Design review of the part built by this model. Coordinates are the model's own, in mm. A direction names the side the tool comes from. Give positions to 0.01 mm unless a question says otherwise; leave off trailing zeros. Loops run counter-clockwise (first coordinate to the right, second up) from the corner with the lowest first, then second, coordinate; pieces in that order, holes last.
from build123d import *

# Parameters (mm, degrees)
ESQUISSE1_R             = 2.05
ESQUISSE1_R_2           = 1.55
ESQUISSE1_R_3           = 3
BOSS_EXTRU_1_DEPTH      = 9
CONG_2_R                = 5
ESQUISSE2_R             = 1.5
ENL_V_MAT_EXTRU_1_DEPTH = 10


with BuildPart() as part:
    # Esquisse1 → Boss.-Extru.1 (new body)
    with BuildSketch(Plane(origin=(0, 0, 0), x_dir=(1, 0, 0), z_dir=(0, 1, 0))):
        Polygon((150, -69), (150, 69), (-149.848840409, 69), (-150, 69), (-150, -69), (-120, -69), (-120, -99), (120, -99), (120, -69), align=None)
        with Locations(Location((-140, 59, 0), (0, 0, 270))):
            Circle(ESQUISSE1_R, mode=Mode.SUBTRACT)
        with Locations(Location((140, 59, 0), (0, 0, 90))):
            Circle(ESQUISSE1_R, mode=Mode.SUBTRACT)
        with Locations(Location((140, -59, 0), (0, 0, 270))):
            Circle(ESQUISSE1_R, mode=Mode.SUBTRACT)
        with Locations(Location((-140, -59, 0), (0, 0, 90))):
            Circle(ESQUISSE1_R, mode=Mode.SUBTRACT)
        with Locations(Location((-48, -83, 0), (0, 0, 270))):
            Circle(ESQUISSE1_R_2, mode=Mode.SUBTRACT)
        with Locations(Location((-104, -83, 0), (0, 0, 270))):
            Circle(ESQUISSE1_R_2, mode=Mode.SUBTRACT)
        with Locations(Location((-48, -64, 0), (0, 0, 270))):
            Circle(ESQUISSE1_R_2, mode=Mode.SUBTRACT)
        with Locations(Location((-104, -64, 0), (0, 0, 270))):
            Circle(ESQUISSE1_R_2, mode=Mode.SUBTRACT)
        with Locations(Location((82.54, -28.63, 0), (0, 0, 270))):
            Circle(ESQUISSE1_R_2, mode=Mode.SUBTRACT)
        with Locations(Location((130.8, -27.36, 0), (0, 0, 270))):
            Circle(ESQUISSE1_R_2, mode=Mode.SUBTRACT)
        with Locations(Location((130.8, 47.57, 0), (0, 0, 270))):
            Circle(ESQUISSE1_R_2, mode=Mode.SUBTRACT)
        with Locations(Location((82.54, 53.92, 0), (0, 0, 270))):
            Circle(ESQUISSE1_R_2, mode=Mode.SUBTRACT)
        with Locations(Location((87.62, 23.44, 0), (0, 0, 270))):
            Circle(ESQUISSE1_R_2, mode=Mode.SUBTRACT)
        with Locations(Location((38, -54, 0), (0, 0, 270))):
            Circle(ESQUISSE1_R_2, mode=Mode.SUBTRACT)
        with Locations(Location((75, -54, 0), (0, 0, 270))):
            Circle(ESQUISSE1_R_2, mode=Mode.SUBTRACT)
        with Locations(Location((75, -91, 0), (0, 0, 270))):
            Circle(ESQUISSE1_R_2, mode=Mode.SUBTRACT)
        with Locations(Location((38, -91, 0), (0, 0, 270))):
            Circle(ESQUISSE1_R_2, mode=Mode.SUBTRACT)
        with Locations(Location((-132.5, 50.5, 0), (0, 0, 270))):
            Circle(ESQUISSE1_R_2, mode=Mode.SUBTRACT)
        with Locations(Location((-132.5, -7.5, 0), (0, 0, 270))):
            Circle(ESQUISSE1_R_2, mode=Mode.SUBTRACT)
        with Locations(Location((-83.5, -7.5, 0), (0, 0, 270))):
            Circle(ESQUISSE1_R_2, mode=Mode.SUBTRACT)
        with Locations(Location((-83.5, 50.5, 0), (0, 0, 270))):
            Circle(ESQUISSE1_R_2, mode=Mode.SUBTRACT)
        with Locations(Location((-55.25, 52, 0), (0, 0, 270))):
            Circle(ESQUISSE1_R_2, mode=Mode.SUBTRACT)
        with Locations(Location((-55.25, -12, 0), (0, 0, 270))):
            Circle(ESQUISSE1_R_2, mode=Mode.SUBTRACT)
        with Locations(Location((55.25, 52, 0), (0, 0, 270))):
            Circle(ESQUISSE1_R_2, mode=Mode.SUBTRACT)
        with Locations(Location((55.25, -12, 0), (0, 0, 270))):
            Circle(ESQUISSE1_R_2, mode=Mode.SUBTRACT)
        with Locations(Location((-24.75, -56.5, 0), (0, 0, 270))):
            Circle(ESQUISSE1_R_2, mode=Mode.SUBTRACT)
        with Locations(Location((24.75, -56.5, 0), (0, 0, 270))):
            Circle(ESQUISSE1_R_2, mode=Mode.SUBTRACT)
        with Locations(Location((27.5, -72.5, 0), (0, 0, 270))):
            Circle(ESQUISSE1_R_3, mode=Mode.SUBTRACT)
        with Locations(Location((85.5, -72.5, 0), (0, 0, 270))):
            Circle(ESQUISSE1_R_3, mode=Mode.SUBTRACT)
        with Locations(Location((-76, -56, 0), (0, 0, 270))):
            Circle(ESQUISSE1_R_3, mode=Mode.SUBTRACT)
        with BuildLine():
            Line((-56, -95.5), (-96, -95.5))
            ThreePointArc((-96, -95.5), (-98.5, -93), (-96, -90.5))
            Line((-96, -90.5), (-56, -90.5))
            ThreePointArc((-56, -90.5), (-53.5, -93), (-56, -95.5))
        make_face(mode=Mode.SUBTRACT)
        with BuildLine():
            Line((-5, 66.5), (5, 66.5))
            ThreePointArc((5, 66.5), (7.5, 64), (5, 61.5))
            Line((5, 61.5), (-5, 61.5))
            ThreePointArc((-5, 61.5), (-7.5, 64), (-5, 66.5))
        make_face(mode=Mode.SUBTRACT)
        with BuildLine():
            Line((-42.5, -35.25), (-42.5, -45.25))
            ThreePointArc((-42.5, -45.25), (-45, -47.75), (-47.5, -45.25))
            Line((-47.5, -45.25), (-47.5, -35.25))
            ThreePointArc((-47.5, -35.25), (-45, -32.75), (-42.5, -35.25))
        make_face(mode=Mode.SUBTRACT)
        with BuildLine():
            Line((42.5, -35.25), (42.5, -45.25))
            ThreePointArc((42.5, -45.25), (45, -47.75), (47.5, -45.25))
            Line((47.5, -45.25), (47.5, -35.25))
            ThreePointArc((47.5, -35.25), (45, -32.75), (42.5, -35.25))
        make_face(mode=Mode.SUBTRACT)
    extrude(amount=BOSS_EXTRU_1_DEPTH)

    # Congé2
    cong_2_edges = [part.edges().sort_by_distance(p)[0] for p in [
        (150, 4.5, -69),
        (150, 4.5, 69),
        (120, 4.5, 69),
        (120, 4.5, 99),
        (-120, 4.5, 99),
        (-120, 4.5, 69),
        (-150, 4.5, 69),
        (-150, 4.5, -69),
    ]]
    fillet(cong_2_edges, radius=CONG_2_R)

    # Esquisse2 → Enlèv. mat.-Extru.1 (cut)
    with BuildSketch(Plane(origin=(0, 9, 0), x_dir=(1, 0, 0), z_dir=(0, 1, 0))):
        with Locations(Location((-7.5, 45, 0), (0, 0, 270))):
            Circle(ESQUISSE2_R)
        with Locations(Location((7.5, 45, 0), (0, 0, 90))):
            Circle(ESQUISSE2_R)
        with Locations(Location((-7.5, 12, 0), (0, 0, 270))):
            Circle(ESQUISSE2_R)
        with Locations(Location((7.5, 12, 0), (0, 0, 90))):
            Circle(ESQUISSE2_R)
        with Locations(Location((-7.5, -21, 0), (0, 0, 270))):
            Circle(ESQUISSE2_R)
        with Locations(Location((7.5, -21, 0), (0, 0, 90))):
            Circle(ESQUISSE2_R)
        with Locations(Location((-7.5, -54, 0), (0, 0, 270))):
            Circle(ESQUISSE2_R)
        with Locations(Location((7.5, -54, 0), (0, 0, 90))):
            Circle(ESQUISSE2_R)
        with Locations(Location((-7.5, -87, 0), (0, 0, 270))):
            Circle(ESQUISSE2_R)
        with Locations(Location((7.5, -87, 0), (0, 0, 90))):
            Circle(ESQUISSE2_R)
        with Locations(Location((-100, 6, 0), (0, 0, 270))):
            Circle(ESQUISSE2_R)
        with Locations(Location((-100, -6, 0), (0, 0, 90))):
            Circle(ESQUISSE2_R)
        with Locations(Location((100, -6, 0), (0, 0, 270))):
            Circle(ESQUISSE2_R)
        with Locations(Location((100, 6, 0), (0, 0, 90))):
            Circle(ESQUISSE2_R)
        with Locations(Location((-83.5, -80.5, 0), (0, 0, 270))):
            Circle(ESQUISSE2_R)
        with Locations(Location((-68.5, -80.5, 0), (0, 0, 90))):
            Circle(ESQUISSE2_R)
        with Locations(Location((-45, -6, 0), (0, 0, 90))):
            Circle(ESQUISSE2_R)
        with Locations(Location((-45, 6, 0), (0, 0, 270))):
            Circle(ESQUISSE2_R)
        with Locations(Location((45, 6, 0), (0, 0, 90))):
            Circle(ESQUISSE2_R)
        with Locations(Location((45, -6, 0), (0, 0, 270))):
            Circle(ESQUISSE2_R)
    extrude(amount=-ENL_V_MAT_EXTRU_1_DEPTH, mode=Mode.SUBTRACT)


solid = part.part
Q1. Wall thickness on line 1 (Z direction, x = 140, y = 6.5); line 2 (X direction, y = 6.5, z = 56.5); line 3 (X direction, y = 5, z = -12): over which ranges is each line inside the solid? List them lowest first.
Results:
line 1: z = -69 to -61.05, -56.95 to 56.95, 61.05 to 69
line 2: x = -150 to -78.96, -73.04 to -26.3, -23.2 to 23.2, 26.3 to 150
line 3: x = -150 to -9, -6 to 6, 9 to 150
Q2. Take a section at B-B (y = 3.25). Give the number of separate pieces and of enclosed holes in the cut face, plus the area to 3 significant figures.
Results:
separate pieces: 1
enclosed holes: 54
area: 47,700 mm2
Q3. Draft analysis for pull direction Z (two halves, no side actions). For faces 5 (the face through (42.5, 4, 40)), 6 (the face through (-150, 4, -1)), 7 (the face through (135, 4, 69)), state which applies: pulls with the +Z half, pulls with the -Z half, needs draft (parallel to the pull), parting line crosses it, or undercut.
Results:
face 5: undercut
face 6: needs draft
face 7: pulls with the +Z half
Q4. Tool access review of faces 1 (the face through (0, 4, -66.5)), 2 (the face through (-135, 4, 69)), 3 (the face through (-2, 4, 99)), 4 (the face through (120, 4, 84)): name each direction out of +Z, -Z, +X, -X, +Y, -Y from which nothing blocks a thin tool from reaching the whole face with its end or side.
Results:
face 1: +Y, -Y
face 2: +Z, -X, +Y, -Y
face 3: +Z, +X, -X, +Y, -Y
face 4: +Z, +X, +Y, -Y
Q5. Take a section at A-A (x = -76). Give the boundary of the cut face in (y, z), plus the area to 3 significant figures.
Results:
outline: (0, -69) - (9, -69) - (9, 53) - (0, 53) - close; (0, 59) - (9, 59) - (9, 90.5) - (0, 90.5) - close; (0, 95.5) - (9, 95.5) - (9, 99) - (0, 99) - close
area: 1,410 mm2
